For this review, take the finished solid that the model builds, in its own axes (mm). Coordinates: 2 decimals unless noted, no trailing zeros. Write each loop counter-clockwise with the first axis right and the second up, starting at its lowest first coordinate (ties: lowest second). Pieces come first, ordered by that corner, then holes.
```python
from build123d import *

# Parameters (mm, degrees)
BOSS_EXTRUDE1_DEPTH  = 23.025
F_1_5MM_DOWEL_HOLE_D = 1.5


with BuildPart() as part:
    # Sketch1 → Boss-Extrude1 (new body)
    with BuildSketch(Plane.XY):
        Polygon((10.746560597, -0.102705017), (12.746560597, 1.897294983), (12.746560597, 5.297294983), (10.746560597, 7.297294983), align=None)
    extrude(amount=BOSS_EXTRUDE1_DEPTH)

    # Ø1.5mm Dowel Hole (through all)
    with Locations(Plane(origin=(14.246560597, -88.102705017, 36.5), x_dir=(0, 0, -1), z_dir=(1, 0, 0))):
        with Locations((0, 91.7), (-25, 91.7), (25, 91.7)):
            Hole(F_1_5MM_DOWEL_HOLE_D / 2)


solid = part.part
```
1) The part is to be moulded in two halves that separate along Y. For faces 1 (the face through (12.747, 2.4, 11.4)), 2 (the face through (11.73, 0.88, 11.35)), 3 (the face through (11.761, 6.283, 11.351)), 4 (the face through (11.733, 4.104, 10.947)), say which applies: pulls with the +Y half, pulls with the -Y half, needs draft (parallel to the pull), parting line crosses it, or undercut.
2) For L1, parallel to Y at x = 11.4, z = 11.5; L2, parallel to Y at x = 12.1, z = 11.5; L3, parallel to Y at x = 11.55, z = 1.75, list the stretches that pass through material, from the lowest coordinate up.
3) Consider section C-C (z = 4.5). Give the boundary of the cut face in (x, y), then the cut area to 3 significant figures.
4) Clearance check with a flat-ended pin moving along its axis: P1, Ø1, axis at y = 6, z = 10.5, coming from the +X side. State where the tip first meets the part, or that it passes through.
5) Consider section D-D (y = 6.5). Give the boundary of the cut face in (x, z) (3 decimals), then the cut area to 3 significant figures.
6) Consider section B-B (x = 11.3). Give the boundary of the cut face in (y, z) (3 decimals).
7) Consider section A-A (z = 11.5). Give the boundary of the cut face in (x, y), then the cut area to 3 significant figures.
Results:
1. face 1: needs draft
1. face 2: pulls with the -Y half
1. face 3: pulls with the +Y half
1. face 4: undercut
2. L1: y = 0.55 to 2.85, 4.35 to 6.64
2. L2: y = 1.25 to 2.85, 4.35 to 5.94
2. L3: y = 0.7 to 6.49
3. outline: (10.75, -0.1) - (12.75, 1.9) - (12.75, 5.3) - (10.75, 7.3) - close
3. area: 10.8 mm2
4. P1: stops at x = 12.54
5. outline: (10.747, 0) - (11.544, 0) - (11.544, 23.025) - (10.747, 23.025) - close
5. area: 18.4 mm2
6. outline: (0.451, 0) - (6.744, 0) - (6.744, 23.025) - (0.451, 23.025) - close; hole circle Ø1.5 at (3.597, 11.5)
7. outline: (10.75, -0.1) - (12.75, 1.9) - (12.75, 2.85) - (10.75, 2.85) - close; (10.75, 4.35) - (12.75, 4.35) - (12.75, 5.3) - (10.75, 7.3) - close
7. area: 7.80 mm2
